```python
from build123d import *

# Parameters (mm, degrees)
SKETCH1_R                  = 28.7655
BOSS_EXTRUDE1_DEPTH        = 19.05
BOSS_EXTRUDE2_DEPTH        = 6.35
FILLET1_R                  = 3.175
SKETCH8_W                  = 50.8
SKETCH8_H                  = 25.4
BOSS_EXTRUDE4_DEPTH        = 38.1
SKETCH5_R                  = 25.5905
CUT_EXTRUDE1_DEPTH         = 26.4
FILLET2_R                  = 0.79375
F_10_32_TAPPED_HOLE1_D     = 4.0386
F_10_32_TAPPED_HOLE1_DEPTH = 6.35
F_0_257_DIAMETER_HOLE1_D   = 6.5278
F_10_32_TAPPED_HOLE2_D     = 4.0386
F_10_32_TAPPED_HOLE2_DEPTH = 16.764
F_10_32_TAPPED_HOLE2_TIP   = 1.213317848


with BuildPart() as part:
    # Sketch1 → Boss-Extrude1 (new body)
    with BuildSketch(Plane(origin=(0, 0, 0), x_dir=(1, 0, 0), z_dir=(0, 1, 0))):
        Circle(SKETCH1_R)
    extrude(amount=BOSS_EXTRUDE1_DEPTH)



with BuildPart() as body_2:
    # Sketch4 → Boss-Extrude2 (new body)
    with BuildSketch(Plane(origin=(0, 19.05, 0), x_dir=(1, 0, 0), z_dir=(0, 1, 0))):
        Polygon((-33.3375, 34.925), (-6.35, 34.925), (-6.35, 44.45), (6.35, 44.45), (6.35, 34.925), (33.3375, 34.925), (33.3375, -34.925), (-33.3375, -34.925), align=None)
    extrude(amount=BOSS_EXTRUDE2_DEPTH)

    # Fillet1
    fillet1_edges = [body_2.edges().sort_by_distance(p)[0] for p in [
        (33.3375, 22.225, 34.925),
        (-33.3375, 22.225, 34.925),
        (-33.3375, 22.225, -34.925),
        (-6.35, 22.225, -34.925),
        (-6.35, 22.225, -44.45),
        (6.35, 22.225, -44.45),
        (6.35, 22.225, -34.925),
        (33.3375, 22.225, -34.925),
    ]]
    fillet(fillet1_edges, radius=FILLET1_R)


with BuildPart() as part_1:
    add(part.part)

    add(body_2.part)  # Boss-Extrude4 merges body 2
    # Sketch8 → Boss-Extrude4 (add)
    with BuildSketch(Plane.XY.offset(47.625)):
        with Locations((0, 12.7)):
            Rectangle(SKETCH8_W, SKETCH8_H)
    extrude(amount=-BOSS_EXTRUDE4_DEPTH)

    # Sketch5 → Cut-Extrude1 (cut, through all)
    with BuildSketch(Plane(origin=(0, 25.4, 0), x_dir=(1, 0, 0), z_dir=(0, 1, 0))):
        Circle(SKETCH5_R)
    extrude(amount=-CUT_EXTRUDE1_DEPTH, mode=Mode.SUBTRACT)

    # Fillet2
    fillet2_edges = [part_1.edges().sort_by_distance(p)[0] for p in [
        (-25.5905, 25.4, 0),
    ]]
    fillet(fillet2_edges, radius=FILLET2_R)

    # #10-32 Tapped Hole1
    with Locations(Plane(origin=(0, 25.4, 0), x_dir=(1, 0, 0), z_dir=(0, 1, 0))):
        with Locations((-30.1625, 30.1625), (30.1625, 30.1625), (30.1625, -30.1625), (-30.1625, -30.1625)):
            Hole(F_10_32_TAPPED_HOLE1_D / 2, depth=F_10_32_TAPPED_HOLE1_DEPTH)

    # F (0.257) Diameter Hole1 (through all)
    with Locations(Plane(origin=(0, 25.4, 0), x_dir=(1, 0, 0), z_dir=(0, 1, 0))):
        with Locations((0, 38.1), (0, -38.1)):
            Hole(F_0_257_DIAMETER_HOLE1_D / 2)

    # #10-32 Tapped Hole2
    with Locations(Plane.XY.offset(47.625)):
        with Locations((-15.875, 19.05), (-15.875, 6.35), (15.875, 6.35), (15.875, 19.05)):
            Hole(F_10_32_TAPPED_HOLE2_D / 2, depth=F_10_32_TAPPED_HOLE2_DEPTH)
            with Locations((0, 0, -(F_10_32_TAPPED_HOLE2_DEPTH + F_10_32_TAPPED_HOLE2_TIP / 2))):  # 118° drill point
                Cone(0, F_10_32_TAPPED_HOLE2_D / 2, F_10_32_TAPPED_HOLE2_TIP, mode=Mode.SUBTRACT)


solid = part_1.part
```
Geometry: final body of the model. Coordinates: model frame, mm. A direction names the side the tool comes from. Coordinates: 2 decimals unless noted, no trailing zeros. Write each loop counter-clockwise with the first axis right and the second up, starting at its lowest first coordinate (ties: lowest second). Pieces come first, ordered by that corner, then holes. Notation, with made-up numbers: M 86,10.5 L 103,10.5 A30 cw 103,37.5 Z; hole C -8.75,83 d3. An arc over 180 degrees is marked long. Use CSV: the item, a comma, the result in double quotes. Start each with the question number.
1. Cut plane C-C on z = 0. Return the cut outline in (x, y).
2. Cut plane B-B on x = 0. Count the separate pieces of the cut face and the enclosed holes in it, plus the area to 3 significant figures.
3. Mould query, pull axis X, two halves, no side actions, for faces 1 (the face through (32.4, 22.3, -34)), 2 (the face through (0.829, 9.392, -28.754)), 3 (the face through (-15, 25.4, 23)), 4 (the face through (0.708, 12.522, 41.286)). Classes: pulls with the +X half, pulls with the -X half, needs draft (parallel to the pull), parting line crosses it, or undercut.
4. First-contact query: P1, Ø1.5, axis at x = -3, y = 12.5, coming from the -Z side; P2, Ø3, axis at x = -22, y = 20.5, coming from the -Z side (3 decimals); P3, Ø12.5, axis at y = 7.5, z = 30.5, coming from the +X side. Flat tips, straight axial feed; report the tip coordinate or a pass-through.
5. Cut plane A-A on z = 38.1. Return the cut outline in (x, y) (3 decimals).
6. Ray query, probe 1 along Z at (x, y) = (0, 12.75) (1 decimal); probe 2 along X at (y, z) = (6.35, 42.5); probe 3 along Y at (x, z) = (17.5, 37). Return the intervals inside material, ascending.
7. Reachability of faces 5 (the face through (-15.44, 4.38, 39.13)), 6 (the face through (20, 22, -34.925)), 7 (the face through (-20, 22, -34.925)) from +Z, -Z, +X, -X, +Y, -Y: full face, straight path, thin tool, end or side. Return the list, or none.
8. Cut plane D-D on y = 11.75. Return the cut outline in (x, z) (1 decimal), plus the area to 3 significant figures.
Entries:
1,outline,"M -33.34,19.05 L -28.77,19.05 L -28.77,0 L -25.59,0 L -25.59,24.61 A0.79 ccw -26.38,25.4 L -33.34,25.4 Z; M 25.59,0 L 28.77,0 L 28.77,19.05 L 33.34,19.05 L 33.34,25.4 L 26.38,25.4 A0.79 ccw 25.59,24.61 Z"
2,separate pieces,"4"
2,enclosed holes,"0"
2,area,"532 mm²"
3,face 1,"pulls with the +X half"
3,face 2,"parting line crosses it"
3,face 3,"needs draft"
3,face 4,"undercut"
4,P1,"z = -28.68"
4,P2,"z = -34.925"
4,P3,"x = 25.4"
5,outline,"M -25.4,0 L -3.264,0 L -3.264,25.4 L -25.4,25.4 Z; M 3.264,0 L 25.4,0 L 25.4,25.4 L 3.264,25.4 Z; hole C -15.875,6.35 d4.039; hole C -15.875,19.05 d4.039; hole C 15.875,6.35 d4.039; hole C 15.875,19.05 d4.039"
6,probe 1,"-28.8 to -25.6, 25.6 to 34.8, 41.4 to 47.6"
6,probe 2,"-25.4 to -17.89, -13.86 to 13.86, 17.89 to 25.4"
6,probe 3,"0 to 5.15, 7.55 to 17.85, 20.25 to 25.4"
7,face 5,"+Z"
7,face 6,"-Z, +X, +Y, -Y"
7,face 7,"-Z, -X, +Y, -Y"
8,outline,"M -25.4,13.5 A28.8 ccw long 25.4,13.5 L 25.4,47.6 L -25.4,47.6 Z; hole C 0,0 d51.2; hole C 0,38.1 d6.5"
8,area,"1,690 mm²"
